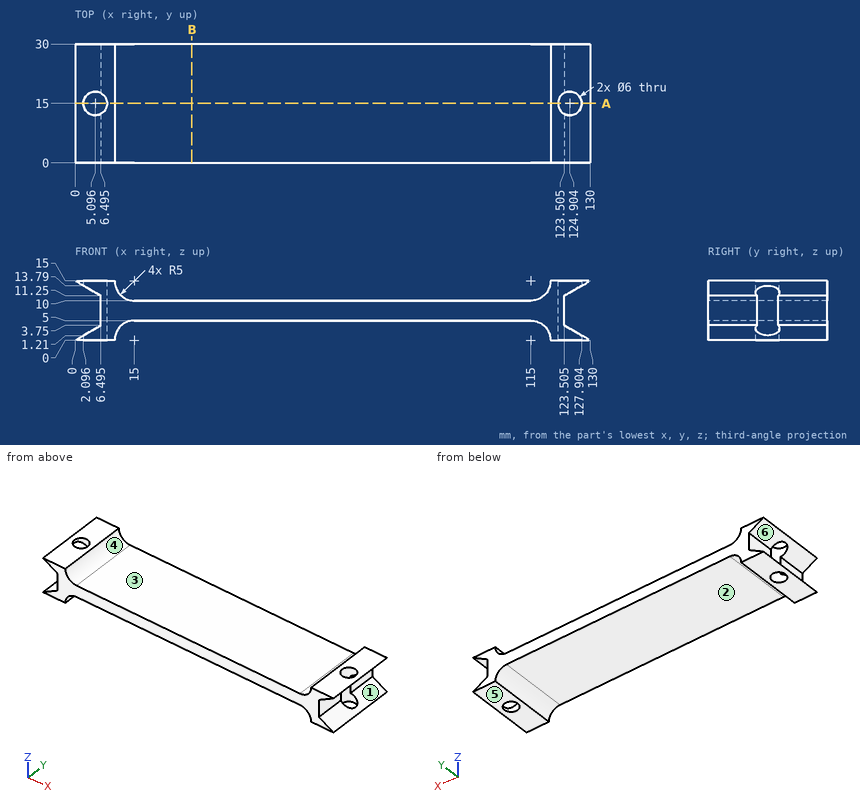
The figure shows three views and two pictorial views of one solid part (mm, origin at its lowest corner). Answer the questions. A direction names the side the tool comes from. Round coordinates to 2 decimals unless told otherwise and drop trailing zeros. Loops run counter-clockwise (first coordinate to the right, second up) from the corner with the lowest first, then second, coordinate; pieces in that order, holes last. Notation, with made-up numbers: M 88.5,-15.5 L 136.5,-15.5 A23 ccw 136.5,17.5 Z; hole C -27,76.25 d11. An arc over 180 degrees is marked long. Use CSV: the item, a comma, the result in double quotes.
Q1. Each of these flat-tipped pins is pushed along its axis until it touches: pin 1 (1 mm diameter, centred on y = 23.5, z = 4, fed in from -X); pin 2 (4 mm diameter, centred on y = 27, z = 2.5, fed in from -X) (1 decimal); pin 3 (1 mm diameter, centred on y = 5, z = 5, fed in from +X) (3 decimals). Where does it stop, or does it pass through?
Determined:
pin 1,"x = 6.06"
pin 2,"x = 0.9"
pin 3,"x = 123.505"
Q2. The mould has two halves that part along X. Classify the marked faces 4, 5 and 6: pulls with the +X half, pulls with the -X half, needs draft (parallel to the pull), parting line crosses it, or undercut.
Determined:
face 4,"undercut"
face 5,"needs draft"
face 6,"pulls with the -X half"
Q3. A tool of negligible diameter and unlimited length cuts with its end or side. For the marked faces 1, 2 and 3, from which of +Z, -Z, +X, -X, +Y, -Y can it reach the whole face along a straight path? Write none if from no direction.
Determined:
face 1,"+X, +Y, -Y"
face 2,"-Z, +Y, -Y"
face 3,"+Z, +Y, -Y"
Q4. Section B-B, the plane x = 29.5 is taken. Determine the outline of the cut face in (y, z), then the cut area to 3 significant figures.
Determined:
outline,"M 0,5 L 30,5 L 30,10 L 0,10 Z"
area,"150 mm2"
Q5. Consider L1, parallel to Z at x = 48.5, y = 10.5; L2, parallel to X at y = 18.5, z = 12.5; L3, parallel to X at y = 14.75, z = 12.25 (1 decimal). Determine where each line is inside the solid, lowest interval first.
Determined:
L1,"5 to 10"
L2,"4.33 to 10.67, 119.33 to 125.67"
L3,"8.1 to 10.8, 119.2 to 121.9"
Q6. Section A-A, the plane y = 15 is taken. Determine the outline of the cut face in (x, z).
Determined:
outline,"M 0,0 L 2.1,0 L 2.1,1.21 Z; M 0,15 L 2.1,13.79 L 2.1,15 Z; M 8.1,0 L 10,0 A5 cw 15,5 L 115,5 A5 cw 120,0 L 121.9,0 L 121.9,15 L 120,15 A5 cw 115,10 L 15,10 A5 cw 10,15 L 8.1,15 Z; M 127.9,0 L 130,0 L 127.9,1.21 Z; M 127.9,13.79 L 130,15 L 127.9,15 Z"
